Verification items for this drawing (mm, ordinates from the low corner). A direction names the side the tool comes from. Coordinates: 2 decimals unless noted, no trailing zeros. Write each loop counter-clockwise with the first axis right and the second up, starting at its lowest first coordinate (ties: lowest second). Pieces come first, ordered by that corner, then holes. Notation, with made-up numbers: (-24, 63) -> (12, 63) arc R20 ccw to (12, 84) -> close; hole circle Ø5 at (-18, 58.25). An arc over 180 degrees is marked (long way). One line per question, with ' | ' between items.
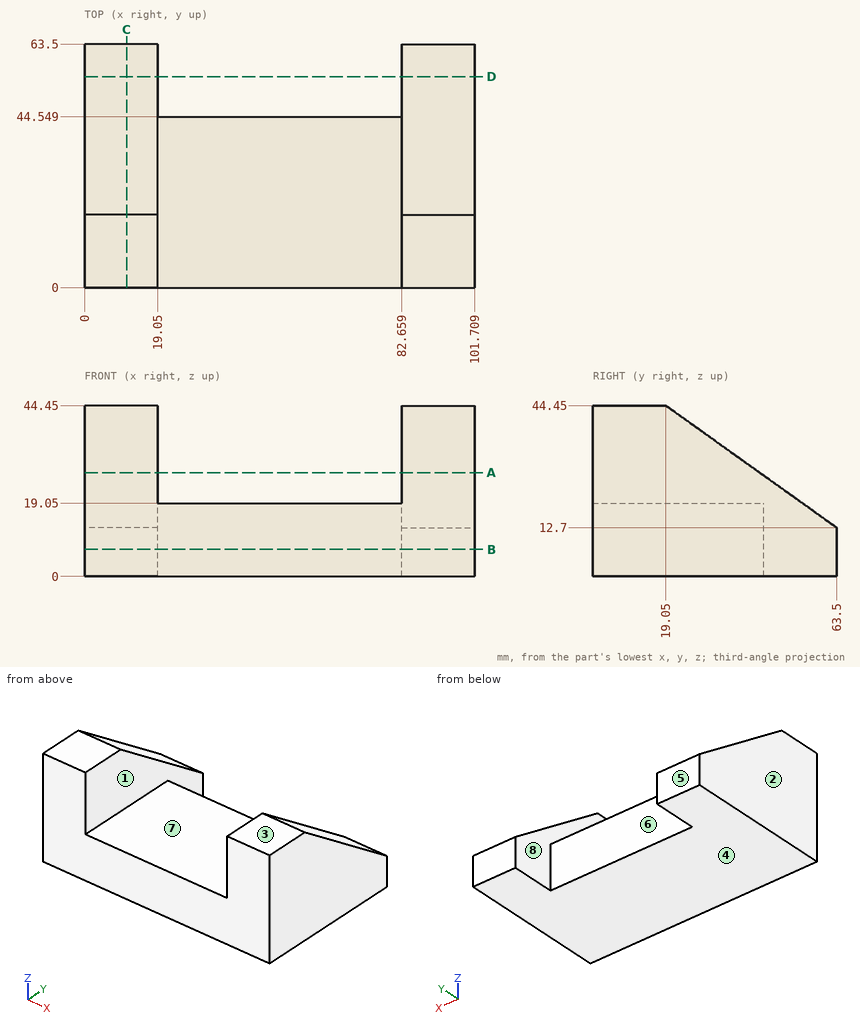
(1) Tool access check on the marked faces 4, 5, 6, 7 and 8. Record the directions out of +Z, -Z, +X, -X, +Y, -Y that give a thin tool (end or side, any length) a straight path to the whole face; none if there is none.
Answers below:
face 4: -Z, +X, -X, +Y, -Y | face 5: +Z, -Z, +X, -X, +Y | face 6: +Z, -Z, +Y | face 7: +Z, +Y, -Y | face 8: +Z, +Y
(2) Cross-section at D-D (y = 55). Record the cut outline in (x, z).
Answers below:
outline: (0, 0) -> (19.05, 0) -> (19.05, 18.77) -> (0, 18.77) -> close; (82.66, 0) -> (101.71, 0) -> (101.71, 18.77) -> (82.66, 18.77) -> close
(3) Depth check by flat-ended pin: P1, Ø5.5, axis at x = 36, z = 6, coming from the +Y side; P2, Ø13.5, axis at x = 66.5, y = 15.5, coming from the +Z side; P3, Ø2, axis at y = 35, z = 16, coming from the -X side. Enter the tip coordinate at first touch or a pass-through.
Answers below:
P1: stops at y = 44.55 | P2: stops at z = 19.05 | P3: stops at x = 0
(4) Cross-section at B-B (z = 7). Record the cut outline in (x, y).
Answers below:
outline: (0, 0) -> (101.71, 0) -> (101.71, 63.5) -> (82.66, 63.5) -> (82.66, 44.55) -> (19.05, 44.55) -> (19.05, 63.5) -> (0, 63.5) -> close
(5) Cross-section at A-A (z = 27). Record the cut outline in (x, y), plus the area to 3 significant figures.
Answers below:
outline: (0, 0) -> (19.05, 0) -> (19.05, 43.48) -> (0, 43.48) -> close; (82.66, 0) -> (101.71, 0) -> (101.71, 43.48) -> (82.66, 43.48) -> close | area: 1,660 mm²
(6) Cross-section at C-C (x = 11). Record the cut outline in (y, z), plus the area to 3 significant figures.
Answers below:
outline: (0, 0) -> (63.5, 0) -> (63.5, 12.7) -> (19.05, 44.45) -> (0, 44.45) -> close | area: 2,120 mm²
(7) Material ranges on line 1 (X direction, y = 14, z = 22); line 2 (Z direction, x = 67.5, y = 19); line 3 (Y direction, x = 62.5, z = 14.5), recorded low to high.
Answers below:
line 1: x = 0 to 19.05, 82.66 to 101.71 | line 2: z = 0 to 19.05 | line 3: y = 0 to 44.55
(8) Draft check along X on the marked faces 1, 2 and 3. Enter one of: pulls with the +X half, pulls with the -X half, needs draft (parallel to the pull), parting line crosses it, or undercut.
Answers below:
face 1: undercut | face 2: pulls with the -X half | face 3: needs draft
